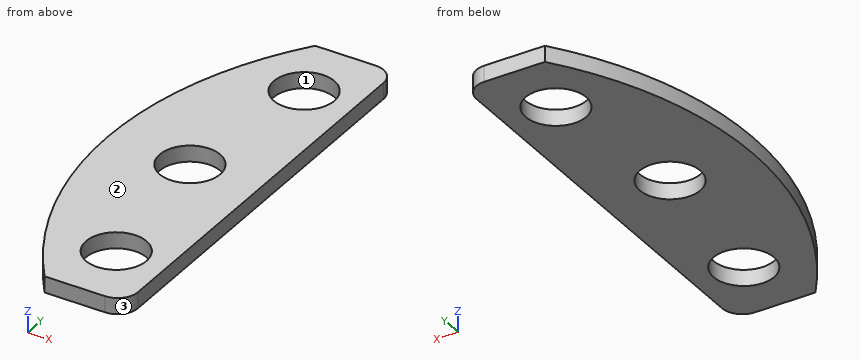
from build123d import *

# Parameters (mm, degrees)
RESSALTO_EXTRUS_O1_DEPTH = 4
ESBO_O2_R                = 7.5
CORTE_EXTRUS_O1_DEPTH    = 10
FILETE1_R                = 5


with BuildPart() as part:
    # Esboço1 → Ressalto-extrusão1 (new body)
    with BuildSketch(Plane.XY):
        with BuildLine():
            Line((-72, -54), (-52, -54))
            Line((-52, -54), (-52, 54))
            Line((-52, 54), (-72, 54))
            ThreePointArc((-72, 54), (-90, 0), (-72, -54))
        make_face()
    extrude(amount=RESSALTO_EXTRUS_O1_DEPTH)

    # Esboço2 → Corte-extrusão1 (cut)
    with BuildSketch(Plane(origin=(0, 0, 0), x_dir=(-1, 0, 0), z_dir=(0, 0, -1))):
        with Locations((69.5, 0)):
            Circle(ESBO_O2_R)
        with Locations((64.5, -37.5)):
            Circle(ESBO_O2_R)
        with Locations((64.5, 37.5)):
            Circle(ESBO_O2_R)
    extrude(amount=-CORTE_EXTRUS_O1_DEPTH, mode=Mode.SUBTRACT)

    # Filete1
    filete1_edges = [part.edges().sort_by_distance(p)[0] for p in [
        (-52, 54, 2),
        (-52, -54, 2),
    ]]
    fillet(filete1_edges, radius=FILETE1_R)


solid = part.part
For this review, take the finished solid that the model builds, in its own axes (mm). Face numbers are marked on the shaded views. Round coordinates to 2 decimals unless told otherwise and drop trailing zeros. Loops run counter-clockwise (first coordinate to the right, second up) from the corner with the lowest first, then second, coordinate; pieces in that order, holes last. Notation, with made-up numbers: (-6, 9) - (31, 9) arc R13 cw to (31, 21) - close; hole circle Ø10 at (-34.75, 65). An arc over 180 degrees is marked (long way). Put each result on its own line as item: value. Start each with the question number.
1. Consider section B-B on z = 0.9. State the section outline as (x, y) points.
2. Consider section A-A on y = 0. State the section outline as (x, z) points, plus the area to 3 significant figures.
3. Consider section D-D on y = -37.5. State the section outline as (x, z) points, plus the area to 3 significant figures.
4. Insertion check: P1, Ø1.5, axis at y = 30, z = 1, coming from the -X side; P2, Ø9, axis at x = -64.5, y = -37.5, coming from the -Z side. Each pin has a flat end and moves straight along its axis. Give the tip position at first contact, or say it passes through.
5. For probe 1 along Y at (x, z) = (-60, 2.6); probe 2 along Y at (x, z) = (-68, 1.4); probe 3 along Y at (x, z) = (-71, 3.2), list the stretches that pass through material, from the lowest coordinate up. Write a range as [from, to].
6. Mouldability with a two-part tool opening along X and no side actions: class the marked faces 1, 2 and 3 as +X half, -X half, draft (parallel to the pull), parting line (faces both ways), or undercut.
7. Consider section C-C on x = -69.5. State the section outline as (y, z) points.
Result sheet:
1. outline: (-72, -54) - (-57, -54) arc R5 ccw to (-52, -49) - (-52, 49) arc R5 ccw to (-57, 54) - (-72, 54) arc R90 ccw to start; hole circle Ø15 at (-69.5, 0); hole circle Ø15 at (-64.5, -37.5); hole circle Ø15 at (-64.5, 37.5)
2. outline: (-90, 0) - (-77, 0) - (-77, 4) - (-90, 4) - close; (-62, 0) - (-52, 0) - (-52, 4) - (-62, 4) - close
2. area: 92.0 mm^2
3. outline: (-81.82, 0) - (-72, 0) - (-72, 4) - (-81.82, 4) - close; (-57, 0) - (-52, 0) - (-52, 4) - (-57, 4) - close
3. area: 59.3 mm^2
4. P1: x = -85.11
4. P2: through
5. probe 1: [-54, -43.5], [-31.5, 31.5], [43.5, 54]
5. probe 2: [-54, -44.13], [-30.87, -7.35], [7.35, 30.87], [44.13, 54]
5. probe 3: [-54, -41.24], [-33.76, -7.35], [7.35, 33.76], [41.24, 54]
6. face 1: undercut
6. face 2: draft
6. face 3: +X half
7. outline: (-54, 0) - (-43.09, 0) - (-43.09, 4) - (-54, 4) - close; (-31.91, 0) - (-7.5, 0) - (-7.5, 4) - (-31.91, 4) - close; (7.5, 0) - (31.91, 0) - (31.91, 4) - (7.5, 4) - close; (43.09, 0) - (54, 0) - (54, 4) - (43.09, 4) - close
